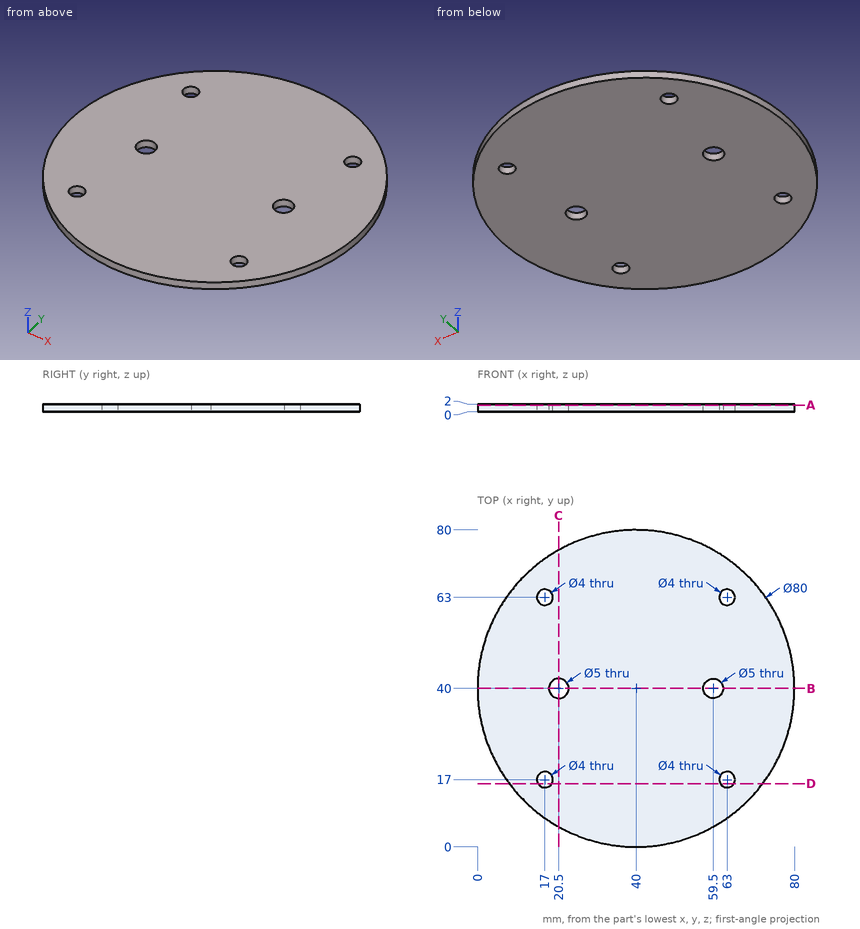
Geometry: see drawing. Coordinates: mm, zero at the bounding-box minimum. Give positions to 0.01 mm unless a question says otherwise; leave off trailing zeros. Write each loop counter-clockwise with the first axis right and the second up, starting at its lowest first coordinate (ties: lowest second). Pieces come first, ordered by that corner, then holes. Notation, with made-up numbers: M 27,0.5 L 61,0.5 A21 cw 61,36.5 Z; hole C 22,-12.75 d2. An arc over 180 degrees is marked long. Answer in a Markdown table with one row per item. Add a question column.
(1) First-contact query: pin 1 (10 mm diameter, centred on x = 32.5, y = 55, fed in from -Z). Flat tip, straight axial feed; report the tip coordinate or a pass-through.
(2) Section D-D on y = 16. Return loops of the section in (x, z).
(3) Ray query, line 1 (X direction, y = 18, z = 1.4); line 2 (X direction, y = 39, z = 0.2); line 3 (Y direction, x = 63, z = 0.55). Return the intervals inside material, ascending.
(4) Section B-B on y = 40. Return loops of the section in (x, z), and give its area (3 significant figures).
(5) Section C-C on x = 20.5. Return loops of the section in (y, z).
(6) Section A-A on z = 1.7. Return loops of the section in (x, y), and give its area (3 significant figures).
Result set:
| question | item | result |
|---|---|---|
| 1 | pin 1 | stops at z = 0 |
| 2 | outline | M 8,0 L 15.27,0 L 15.27,2 L 8,2 Z; M 18.73,0 L 61.27,0 L 61.27,2 L 18.73,2 Z; M 64.73,0 L 72,0 L 72,2 L 64.73,2 Z |
| 3 | line 1 | x = 6.59 to 15.27, 18.73 to 61.27, 64.73 to 73.41 |
| 3 | line 2 | x = 0.01 to 18.21, 22.79 to 57.21, 61.79 to 79.99 |
| 3 | line 3 | y = 7.27 to 15, 19 to 61, 65 to 72.73 |
| 4 | outline | M 0,0 L 18,0 L 18,2 L 0,2 Z; M 23,0 L 57,0 L 57,2 L 23,2 Z; M 62,0 L 80,0 L 80,2 L 62,2 Z |
| 4 | area | 140 mm^2 |
| 5 | outline | M 5.08,0 L 37.5,0 L 37.5,2 L 5.08,2 Z; M 42.5,0 L 74.92,0 L 74.92,2 L 42.5,2 Z |
| 6 | outline | C 40,40 d80; hole C 17,17 d4; hole C 17,63 d4; hole C 20.5,40 d5; hole C 59.5,40 d5; hole C 63,17 d4; hole C 63,63 d4 |
| 6 | area | 4,940 mm^2 |
